Verification items for the finished model (mm, model axes). Face numbers are marked on the shaded views. A direction names the side the tool comes from. Round coordinates to 2 decimals unless told otherwise and drop trailing zeros. Write each loop counter-clockwise with the first axis right and the second up, starting at its lowest first coordinate (ties: lowest second). Pieces come first, ordered by that corner, then holes. Notation, with made-up numbers: M 70.25,57 L 119.25,57 A11 ccw 119.25,71 Z; hole C -7,56 d4. An arc over 180 degrees is marked long. Write each question's results on one line, items separated by ' | '.
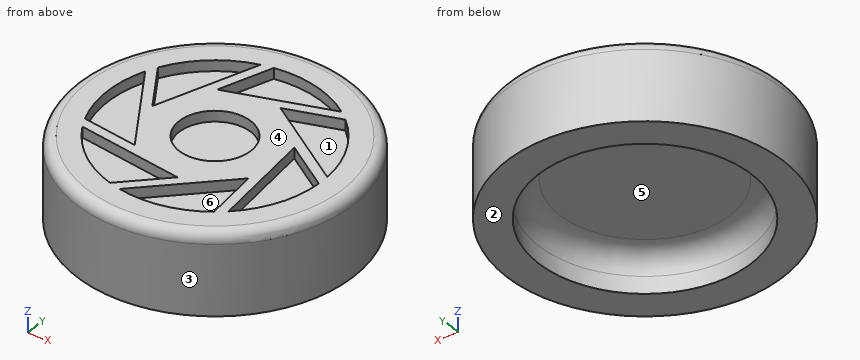
Autodesk Inventor part; units mm, degrees
ref_plane "YZ Plane" through (0, 0, 0) normal (1, 0, 0) x (0, 1, 0)
ref_plane "XZ Plane" through (0, 0, 0) normal (0, 1, 0) x (-1, 0, 0)
ref_plane "XY Plane" through (0, 0, 0) normal (0, 0, 1) x (1, 0, 0)
sketch "Sketch1" plane through (0, 0, 0) normal (0, 0, 1) x (1, 0, 0)
  circle A0 centre (0, 0) radius 6.5
  circle A1 centre (0, 0) radius 5
  point P0 (0, 0)
  dimension "d0" = 1.5
extrude "Extrusion1" add sketch "Sketch1" against normal blind 2.8
sketch "Sketch2" plane through (0, 0, 0) normal (0, 0, 1) x (1, 0, 0)
  circle A0 centre (0, 0) radius 6.5
  point P0 (0, 0)
extrude "Extrusion2" add sketch "Sketch2" along normal mid plane 2
fillet "Fillet1" radius 0.5 1 edges at (-6.5, 0, 1)
sketch "Sketch3" plane through (0, 0, 1) normal (0, 0, 1) x (1, 0, 0)
  line L0 (-1.7757, 2.5328) -> (2.8763, 4.1461)
  arc A0 (2.8763, 4.1461) -> (-0.9181, 4.9618) centre (0, 0) ccw
  line L1 (-0.9181, 4.9618) -> (-1.7757, 2.5328)
  line L2 (0.8731, 2.9674) -> (5.0349, 0.3362)
  arc A1 (5.0349, 0.3362) -> (3.3069, 3.8115) centre (0, 0) ccw
  line L3 (3.3069, 3.8115) -> (0.8731, 2.9674)
  line L4 (2.8644, 1.1676) -> (3.4021, -3.7268)
  arc A2 (3.4021, -3.7268) -> (5.0417, -0.209) centre (0, 0) ccw
  line L5 (5.0417, -0.209) -> (2.8644, 1.1676)
  circle A3 centre (0, 0) radius 1.682
  line L6 (2.6988, -1.5115) -> (-0.7925, -4.9834)
  arc A4 (-0.7925, -4.9834) -> (2.9801, -4.0721) centre (0, 0) ccw
  line L7 (2.9801, -4.0721) -> (2.6988, -1.5115)
  line L8 (0.5009, -3.0524) -> (-4.3904, -2.4875)
  arc A5 (-4.3904, -2.4875) -> (-1.3257, -4.8688) centre (0, 0) ccw
  line L9 (-1.3257, -4.8688) -> (0.5009, -3.0524)
  line L10 (-2.0741, -2.2947) -> (-4.6821, 1.8816)
  arc A6 (-4.6821, 1.8816) -> (-4.6331, -1.9992) centre (0, 0) ccw
  line L11 (-4.6331, -1.9992) -> (-2.0741, -2.2947)
  line L12 (-3.0873, 0.1909) -> (-1.4482, 4.8338)
  arc A7 (-1.4482, 4.8338) -> (-4.4518, 2.3758) centre (0, 0) ccw
  line L13 (-4.4518, 2.3758) -> (-3.0873, 0.1909)
  point P0 (0, 0)
extrude "Extrusion3" cut sketch "Sketch3" against normal blind 0.5
fillet "Fillet2" radius 1 1 edges at (-5, 0, -1)
properties part number "bottom-cap"
1) Sectioned sample at B-B, the plane y = 0. Record the cut outline in (x, z).
Calculated:
outline: M -6.5,-2.8 L -5,-2.8 L -5,-2 A1 cw -4,-1 L 4,-1 A1 cw 5,-2 L 5,-2.8 L 6.5,-2.8 L 6.5,0.5 A0.5 ccw 6,1 L 4.71,1 L 4.71,0.5 L 2.99,0.5 L 2.99,1 L 1.68,1 L 1.68,0.5 L -1.68,0.5 L -1.68,1 L -3.51,1 L -3.51,0.5 L -5.05,0.5 L -5.05,1 L -6,1 A0.5 ccw -6.5,0.5 Z
2) Draft check along X on the marked faces 1, 2 and 3. Enter one of: pulls with the +X half, pulls with the -X half, needs draft (parallel to the pull), parting line crosses it, or undercut.
Calculated:
face 1: undercut | face 2: needs draft | face 3: parting line crosses it
3) Depth check by flat-ended pin: P1, Ø1.5, axis at y = -3, z = -0.5, coming from the -X side; P2, Ø4, axis at x = 2, y = -3, coming from the +Z side; P3, Ø2, axis at x = 0, y = 0, coming from the +Z side; P4, Ø1, axis at x = 2, z = -2, coming from the -Y side. Enter the tip coordinate at first touch or a pass-through.
Calculated:
P1: stops at x = -6.1 | P2: stops at z = 1 | P3: stops at z = 0.5 | P4: stops at y = -6.32
4) Sectioned sample at D-D, the plane z = -0.3. Record the cut outline in (x, y), and give its area (3 significant figures).
Calculated:
outline: C 0,0 d13 | area: 133 mm²
5) Sectioned sample at A-A, the plane z = -2.2. Record the cut outline in (x, y).
Calculated:
outline: C 0,0 d13; hole C 0,0 d10
6) Material ranges on line 1 (Y direction, x = 0, z = -2.4); line 2 (Y direction, x = 0, z = 0.7); line 3 (Y direction, x = 0, z = 0.85), recorded low to high. Write a range as [from, to].
Calculated:
line 1: y = [-6.5, -5], [5, 6.5] | line 2: y = [-6.46, -5.05], [-4.2, -3.55], [-2.99, -1.68], [1.68, 3.15], [5.05, 6.46] | line 3: y = [-6.36, -5.05], [-4.2, -3.55], [-2.99, -1.68], [1.68, 3.15], [5.05, 6.36]
7) Access from +Z, -Z, +X, -X, +Y, -Y to the whole of each face (thin tool, end or side, straight path). Record for the marked faces 4, 5 and 6.
Calculated:
face 4: +Z, +X, -X, +Y, -Y | face 5: -Z | face 6: +Z
8) Sectioned sample at C-C, the plane x = 0. Record the cut outline in (y, z).
Calculated:
outline: M -6.5,-2.8 L -5,-2.8 L -5,-2 A1 cw -4,-1 L 4,-1 A1 cw 5,-2 L 5,-2.8 L 6.5,-2.8 L 6.5,0.5 A0.5 ccw 6,1 L 5.05,1 L 5.05,0.5 L 3.15,0.5 L 3.15,1 L 1.68,1 L 1.68,0.5 L -1.68,0.5 L -1.68,1 L -2.99,1 L -2.99,0.5 L -3.55,0.5 L -3.55,1 L -4.2,1 L -4.2,0.5 L -5.05,0.5 L -5.05,1 L -6,1 A0.5 ccw -6.5,0.5 Z
